The model under review builds one solid part; all positions refer to its coordinate system, in mm. Face numbers are marked on the shaded views. A direction names the side the tool comes from. Round coordinates to 2 decimals unless told otherwise and drop trailing zeros. Write each loop counter-clockwise with the first axis right and the second up, starting at its lowest first coordinate (ties: lowest second). Pieces come first, ordered by that corner, then holes. Notation, with made-up numbers: (43, 72.5) -> (68, 72.5) arc R22 ccw to (68, 111.5) -> close; hole circle Ø1 at (0, 78.25). An arc over 180 degrees is marked (long way). Answer in a Markdown table with one row per item. Add a question column.
```python
from build123d import *

# Parameters (mm, degrees)
SKETCH1_R               = 10.5
BOSS_EXTRUDE1_DEPTH     = 2.5
SKETCH2_R               = 4.5
SKETCH2_R_2             = 3
BOSS_EXTRUDE2_DEPTH     = 3.5
SKETCH4_R               = 1.5
CUT_EXTRUDE1_DEPTH      = 3.5
CUT_EXTRUDE2_DEPTH      = 16.256146302
CUT_EXTRUDE2_DEPTH_BACK = 16.256146302
SKETCH5_R               = 1.9
CHAMFER1_SIZE           = 0.5


with BuildPart() as part:
    # Sketch1 → Boss-Extrude1 (new body)
    with BuildSketch(Plane(origin=(0, 0, 0), x_dir=(1, 0, 0), z_dir=(0, 1, 0))):
        with Locations(Location((0, 0, 0), (0, 0, 270))):
            Circle(SKETCH1_R)
    extrude(amount=BOSS_EXTRUDE1_DEPTH)

    # Sketch2 → Boss-Extrude2 (add)
    with BuildSketch(Plane(origin=(0, 2.5, 0), x_dir=(1, 0, 0), z_dir=(0, 1, 0))):
        with Locations(Location((0, 0, 0), (0, 0, 270))):
            Circle(SKETCH2_R)
        with Locations(Location((0, 0, 0), (0, 0, 270))):
            Circle(SKETCH2_R_2, mode=Mode.SUBTRACT)
    extrude(amount=BOSS_EXTRUDE2_DEPTH)

    # Sketch4 → Cut-Extrude1 (cut)
    with BuildSketch(Plane(origin=(0, 2.5, 0), x_dir=(1, 0, 0), z_dir=(0, 1, 0))):
        with Locations(Location((0, 0, 0), (0, 0, 270))):
            Circle(SKETCH4_R)
    extrude(amount=-CUT_EXTRUDE1_DEPTH, mode=Mode.SUBTRACT)

    # Sketch5 → Cut-Extrude2 (cut, two sides: drawn at the far end of the back side and taken through both)
    with BuildSketch(Plane(origin=(0, 2.5, 0), x_dir=(1, 0, 0), z_dir=(0, 1, 0)).offset(-CUT_EXTRUDE2_DEPTH_BACK)):
        with Locations(Location((-7.1, 0, 0), (0, 0, 270))):
            Circle(SKETCH5_R)
        with Locations(Location((7.1, 0, 0), (0, 0, 270))):
            Circle(SKETCH5_R)
    extrude(amount=CUT_EXTRUDE2_DEPTH + CUT_EXTRUDE2_DEPTH_BACK, mode=Mode.SUBTRACT)

    # Chamfer1
    chamfer1_edges = [part.edges().sort_by_distance(p)[0] for p in [
        (0, 2.5, -4.5),
    ]]
    chamfer(chamfer1_edges, length=CHAMFER1_SIZE)


solid = part.part
```
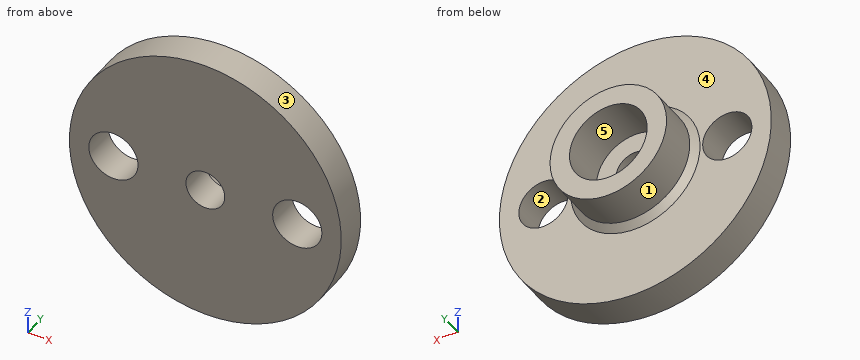
1. For L1, parallel to X at y = 1.4, z = 0; L2, parallel to X at y = 4.5, z = 0; L3, parallel to Y at x = 7.5, z = 4, list the stretches that pass through material, from the lowest coordinate up.
2. Add section B-B on z = 0. Write out the cut boundary in (x, y), plus the area to 4 significant figures.
3. Tool access review of the marked faces 1 and 2: name each direction out of +Z, -Z, +X, -X, +Y, -Y from which nothing blocks a thin tool from reaching the whole face with its end or side.
4. Add section D-D on x = -6.75. Write out the cut boundary in (y, z), plus the area to 3 significant figures.
5. Insertion check: pin 1 Ø2 at (x, y) = (5.5, 2.5) entering from -Z; pin 2 Ø1 at (y, z) = (5.5, 2) entering from +X; pin 3 Ø5 at (x, z) = (0, 0) entering from +Y. Each pin has a flat end and moves straight along its axis. Give the tip position at first contact, or say it passes through.
6. Add section A-A on x = 0. Write out the cut boundary in (y, z).
7. Add section C-C on y = 4.7. Write out the cut boundary in (x, z).
8. Mouldability with a two-part tool opening along X and no side actions: class the marked faces 3, 4 and 5 as pulls with the +X half, pulls with the -X half, needs draft (parallel to the pull), parting line crosses it, or undercut.
Filled in:
| question | item | result |
|---|---|---|
| 1 | L1 | -10.5 to -9, -5.2 to -1.5, 1.5 to 5.2, 9 to 10.5 |
| 1 | L2 | -4.5 to -3, 3 to 4.5 |
| 1 | L3 | 0 to 2.5 |
| 2 | outline | (-10.5, 0) -> (-9, 0) -> (-9, 2.5) -> (-10.5, 2.5) -> close; (-5.2, 0) -> (-1.5, 0) -> (-1.5, 2.5) -> (-3, 2.5) -> (-3, 6) -> (-4.5, 6) -> (-4.5, 3) -> (-5, 2.5) -> (-5.2, 2.5) -> close; (1.5, 0) -> (5.2, 0) -> (5.2, 2.5) -> (5, 2.5) -> (4.5, 3) -> (4.5, 6) -> (3, 6) -> (3, 2.5) -> (1.5, 2.5) -> close; (9, 0) -> (10.5, 0) -> (10.5, 2.5) -> (9, 2.5) -> close |
| 2 | area | 36.75 mm² |
| 3 | face 1 | +Y |
| 3 | face 2 | +Y, -Y |
| 4 | outline | (0, -8.04) -> (2.5, -8.04) -> (2.5, -1.87) -> (0, -1.87) -> close; (0, 1.87) -> (2.5, 1.87) -> (2.5, 8.04) -> (0, 8.04) -> close |
| 4 | area | 30.9 mm² |
| 5 | pin 1 | z = -9.49 |
| 5 | pin 2 | x = 4.24 |
| 5 | pin 3 | y = 2.5 |
| 6 | outline | (0, -10.5) -> (2.5, -10.5) -> (2.5, -5) -> (3, -4.5) -> (6, -4.5) -> (6, -3) -> (2.5, -3) -> (2.5, -1.5) -> (0, -1.5) -> close; (0, 1.5) -> (2.5, 1.5) -> (2.5, 3) -> (6, 3) -> (6, 4.5) -> (3, 4.5) -> (2.5, 5) -> (2.5, 10.5) -> (0, 10.5) -> close |
| 7 | outline | circle Ø9 at (0, 0); hole circle Ø6 at (0, 0) |
| 8 | face 3 | parting line crosses it |
| 8 | face 4 | needs draft |
| 8 | face 5 | undercut |
